The model under review builds one solid part; all positions refer to its coordinate system, in mm. A direction names the side the tool comes from. Round coordinates to 2 decimals unless told otherwise and drop trailing zeros. Order: outer loops, then holes, each group sorted by start corner. A loop starts at its lowest first (then second) coordinate and runs counter-clockwise, first axis right, second up. Notation, with made-up numbers: (66.25, 56.25) -> (124.25, 56.25) arc R19 cw to (124.25, 85.25) -> close; hole circle Ø8 at (46, 54). An arc over 180 degrees is marked (long way). Put each result on its own line as item: value. Start each with the question number.
from build123d import *

# Parameters (mm, degrees)
SKETCH_1_W      = 355
SKETCH_1_H      = 215
EXTRUDE_1_DEPTH = 7
SKETCH_2_R      = 3
SKETCH_2_R_2    = 0.5
EXTRUDE_2_DEPTH = 7


with BuildPart() as part:
    # 草图1 → 凸台-拉伸1 (new body)
    with BuildSketch(Plane.XY):
        with Locations((177.5, -107.5)):
            Rectangle(SKETCH_1_W, SKETCH_1_H)
    extrude(amount=EXTRUDE_1_DEPTH)

    # 草图2 → 凸台-拉伸2 (add)
    with BuildSketch(Plane(origin=(0, 0, 0), x_dir=(-1, 0, 0), z_dir=(0, 0, -1))):
        Polygon((-177.5, -175), (-107.5, -175), (-107.5, -125), (-107.5, -105), (-247.5, -105), (-247.5, -175), align=None)
        with Locations((-177.5, -135)):
            Circle(SKETCH_2_R, mode=Mode.SUBTRACT)
        with Locations((-192.5, -135)):
            Circle(SKETCH_2_R_2, mode=Mode.SUBTRACT)
    extrude(amount=EXTRUDE_2_DEPTH)


solid = part.part
Q1. Clearance check with flat-ended pins moving along their axes: pin 1 Ø4 at (x, z) = (171.5, -5) entering from +Y; pin 2 Ø3 at (x, y) = (176.5, -135.5) entering from -Z; pin 3 Ø2 at (x, z) = (153, -4) entering from -Y. State where each tip first meets the part, or that it passes through.
Q2. Take a section at B-B on x = 123.5. Give the boundary of the cut face in (y, z).
Q3. Take a section at D-D on x = 54. Give the boundary of the cut face in (y, z), and give its area (4 significant figures).
Q4. Wall thickness on probe 1 along X at (y, z) = (-135, -2); probe 2 along Y at (x, z) = (192.5, -1.75); probe 3 along Y at (x, z) = (177.5, -3.25): over which ranges is each line inside the solid? List them lowest first. Write a range as [from, to].
Q5. Take a section at C-C on y = -74.5. Give the boundary of the cut face in (x, z), and give its area (4 significant figures).
Q6. Take a section at A-A on z = -3.75. Give the boundary of the cut face in (x, y), and give its area (3 significant figures).
Q7. For faces 1 (the face through (178, -175, -3)), 2 (the face through (177, -105, -3)), 3 (the face through (0, -109, 3)), 4 (the face through (247.5, -140, -3)), 5 (the face through (107.5, -140, -3)), list the 3-axis set-ups (+Z, -Z, +X, -X, +Y, -Y) from which the entire face can be reached by the end or side of a thin tool; tool diameter is ignored.
Calculated:
1. pin 1: stops at y = -105
1. pin 2: stops at z = 0
1. pin 3: stops at y = -175
2. outline: (-215, 0) -> (-175, 0) -> (-175, -7) -> (-105, -7) -> (-105, 0) -> (0, 0) -> (0, 7) -> (-215, 7) -> close
3. outline: (-215, 0) -> (0, 0) -> (0, 7) -> (-215, 7) -> close
3. area: 1,505 mm²
4. probe 1: x = [107.5, 174.5], [180.5, 192], [193, 247.5]
4. probe 2: y = [-175, -135.5], [-134.5, -105]
4. probe 3: y = [-175, -138], [-132, -105]
5. outline: (0, 0) -> (355, 0) -> (355, 7) -> (0, 7) -> close
5. area: 2,485 mm²
6. outline: (107.5, -175) -> (247.5, -175) -> (247.5, -105) -> (107.5, -105) -> close; hole circle Ø6 at (177.5, -135); hole circle Ø1 at (192.5, -135)
6. area: 9,770 mm²
7. face 1: -Z, +X, -X, -Y
7. face 2: -Z, +X, -X, +Y
7. face 3: +Z, -Z, -X, +Y, -Y
7. face 4: -Z, +X, +Y, -Y
7. face 5: -Z, -X, +Y, -Y
